Geometry: final body of the model. Coordinates: model frame, mm. Coordinates: 2 decimals unless noted, no trailing zeros. Loops run counter-clockwise (first coordinate to the right, second up) from the corner with the lowest first, then second, coordinate; pieces in that order, holes last. Notation, with made-up numbers: (51.5, 13.25) - (81.5, 13.25) arc R7 cw to (81.5, 20.25) - close; hole circle Ø7 at (-20, 34). An arc over 180 degrees is marked (long way). Return JSON: item names as keys, results as strings.
from build123d import *

# Parameters (mm, degrees)
SKETCH1_W           = 30
SKETCH1_H           = 380
BOSS_EXTRUDE1_DEPTH = 5.2
SKETCH2_W           = 20
SKETCH2_H           = 4.9
CUT_EXTRUDE1_DEPTH  = 10
CHAMFER1_SIZE       = 3


with BuildPart() as part:
    # Sketch1 → Boss-Extrude1 (new body)
    with BuildSketch(Plane(origin=(0, 0, 0), x_dir=(1, 0, 0), z_dir=(0, 1, 0))):
        with Locations((15, 190)):
            Rectangle(SKETCH1_W, SKETCH1_H)
    extrude(amount=BOSS_EXTRUDE1_DEPTH)

    # Sketch2 → Cut-Extrude1 (cut)
    with BuildSketch(Plane(origin=(0, 5.2, 0), x_dir=(1, 0, 0), z_dir=(0, 1, 0))):
        with Locations((10, 367.55)):
            Rectangle(SKETCH2_W, SKETCH2_H)
        with Locations((10, 12.45)):
            Rectangle(SKETCH2_W, SKETCH2_H)
    extrude(amount=-CUT_EXTRUDE1_DEPTH, mode=Mode.SUBTRACT)

    # Chamfer1
    chamfer1_edges = [part.edges().sort_by_distance(p)[0] for p in [
        (0, 2.6, -365.1),
        (0, 2.6, -370),
        (0, 2.6, -10),
        (0, 2.6, -14.9),
    ]]
    chamfer(chamfer1_edges, length=CHAMFER1_SIZE)


solid = part.part
Item 1: Section query B-B, the plane y = 1.6. Return loops of the section in (x, z), and give its area (3 significant figures).
Worked out:
{"outline": "(0, -380) - (30, -380) - (30, 0) - (0, 0) - (0, -7) - (3, -10) - (20, -10) - (20, -14.9) - (3, -14.9) - (0, -17.9) - (0, -362.1) - (3, -365.1) - (20, -365.1) - (20, -370) - (3, -370) - (0, -373) - close", "area": "11,200 mm^2"}
Item 2: First-contact query: pin 1 Ø1.5 at (y, z) = (2, -367) entering from -X; pin 2 Ø2.5 at (x, y) = (7.5, 2) entering from +Z. Flat tips, straight axial feed; report the tip coordinate or a pass-through.
Worked out:
{"pin 1": "x = 20", "pin 2": "z = 0"}
Item 3: Ray query, probe 1 along Z at (x, y) = (14.5, 1.45). Return the intervals inside material, ascending. Write a range as from..to.
Worked out:
{"probe 1": "-380..-370, -365.1..-14.9, -10..0"}
Item 4: Section query A-A, the plane x = 11.5. Return loops of the section in (y, z).
Worked out:
{"outline": "(0, -380) - (5.2, -380) - (5.2, -370) - (0, -370) - close; (0, -365.1) - (5.2, -365.1) - (5.2, -14.9) - (0, -14.9) - close; (0, -10) - (5.2, -10) - (5.2, 0) - (0, 0) - close"}
